from build123d import *

# Parameters (mm, degrees)
DODANIE_WYCI_GNI_CIE1_DEPTH       = 3
SZKIC2_W                          = 10
SZKIC2_H                          = 14
SZKIC2_R                          = 2.1
DODANIE_WYCI_GNI_CIE2_DEPTH       = 4
SFAZOWANIE1_SIZE                  = 4
SZYK_LINIOWY1_COUNT               = 2
SZYK_LINIOWY1_PITCH               = 100
SFAZOWANIE1_OF_SZYK_LINIOWY1_SIZE = 4


with BuildPart() as part:
    # Szkic1 → Dodanie-wyciągnięcie1 (new body)
    with BuildSketch(Plane.XY):
        Polygon((0, 0), (187, 0), (187, 30), (15, 30), align=None)
    extrude(amount=DODANIE_WYCI_GNI_CIE1_DEPTH)

    # Szkic2 → Dodanie-wyciągnięcie2 (add)
    with BuildSketch(Plane(origin=(0, 0, 0), x_dir=(-1, 0, 0), z_dir=(0, 0, -1))):
        with Locations((-155, -2)):
            Rectangle(SZKIC2_W, SZKIC2_H)
        with Locations((-155, -5)):
            Circle(SZKIC2_R, mode=Mode.SUBTRACT)
    dodanie_wyci_gni_cie2 = extrude(amount=DODANIE_WYCI_GNI_CIE2_DEPTH)

    # Sfazowanie1
    sfazowanie1_edges = [part.edges().sort_by_distance(p)[0] for p in [
        (160, 2.5, 0),
        (155, 5, 0),
        (150, 2.5, 0),
    ]]
    chamfer(sfazowanie1_edges, length=SFAZOWANIE1_SIZE - 0.0001)  # a hair under: the kernel refuses the full size

    # Szyk liniowy1: Dodanie-wyciągnięcie2 ×2
    with Locations(*[(-i * SZYK_LINIOWY1_PITCH, 0, 0) for i in range(1, SZYK_LINIOWY1_COUNT)]):
        add(dodanie_wyci_gni_cie2)

    # Sfazowanie1 of Szyk liniowy1
    sfazowanie1_of_szyk_liniowy1_edges = [part.edges().sort_by_distance(p)[0] for p in [
        (60, 2.5, 0),
        (55, 5, 0),
        (50, 2.5, 0),
    ]]
    chamfer(sfazowanie1_of_szyk_liniowy1_edges, length=SFAZOWANIE1_OF_SZYK_LINIOWY1_SIZE - 0.0001)  # a hair under: the kernel refuses the full size


solid = part.part
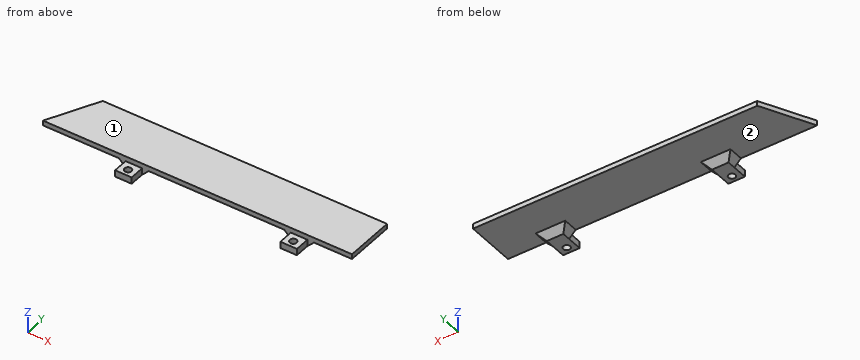
Could you check a few things on this model? Use its own coordinates, in mm. Face numbers are marked on the shaded views. A direction names the side the tool comes from. Coordinates: 2 decimals unless noted, no trailing zeros. Write each loop counter-clockwise with the first axis right and the second up, starting at its lowest first coordinate (ties: lowest second). Pieces come first, ordered by that corner, then holes. Notation, with made-up numbers: (-16, -38) - (18, -38) arc R26 cw to (18, -11) - close; hole circle Ø9 at (-32.5, 37.25). An arc over 180 degrees is marked (long way). Put each result on its own line as item: value. Start each with the question number.
Q1. Please list where these lines run through material, in increasing order: L1, parallel to Z at x = 115, y = 8; L2, parallel to Y at x = 131, z = 0.5; L3, parallel to Y at x = 155, z = -1.9.
Q2. I want a section at D-D on y = 7. Write out the boundary of the cut face in (x, z).
Q3. I want a section at C-C on z = -2.5. Write out the boundary of the cut face in (x, y), plus the area to 3 significant figures.
Q4. I want a section at B-B on y = -5. Write out the boundary of the cut face in (x, z).
Q5. I'm going to push flat-ended pins straight in: P1, Ø1.5, axis at x = 159.5, z = 1, coming from the -Y side; P2, Ø3.5, axis at x = 155, y = -5, coming from the +Z side; P3, Ø3, axis at y = -2.5, z = -1.5, coming from the -X side; P4, Ø9, axis at x = 135.5, y = 16.5, coming from the -Z side. Where does each tip first touch, or does it pass through?
Q6. Which directions (+Z, -Z, +X, -X, +Y, -Y) give clear straight access to the entire face, cutting with the end or side of a thin tool? Please do the marked faces 1 and 2.
Checks:
1. L1: 0 to 3
1. L2: 0 to 30
1. L3: -9 to -7.1, -2.9 to 7.1
2. outline: (3.5, 0) - (46, 0) - (48, -2) - (62, -2) - (64, 0) - (146, 0) - (148, -2) - (162, -2) - (164, 0) - (187, 0) - (187, 3) - (3.5, 3) - close
3. outline: (48.5, 0) - (50, 0) - (50, -9) - (60, -9) - (60, 0) - (61.5, 0) - (61.5, 6.5) - (48.5, 6.5) - close; (148.5, 0) - (150, 0) - (150, -9) - (160, -9) - (160, 0) - (161.5, 0) - (161.5, 6.5) - (148.5, 6.5) - close; hole circle Ø4.2 at (55, -5); hole circle Ø4.2 at (155, -5)
3. area: 321 mm²
4. outline: (50, -4) - (52.9, -4) - (52.9, 0) - (50, 0) - close; (57.1, -4) - (60, -4) - (60, 0) - (57.1, 0) - close; (150, -4) - (152.9, -4) - (152.9, 0) - (150, 0) - close; (157.1, -4) - (160, -4) - (160, 0) - (157.1, 0) - close
5. P1: y = 0
5. P2: through
5. P3: x = 50
5. P4: z = 0
6. face 1: +Z, +X, -X, +Y, -Y
6. face 2: -Z, +Y
